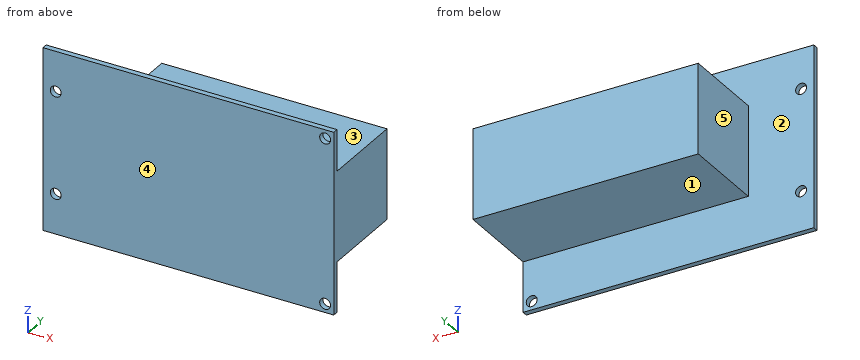
from build123d import *

# Parameters (mm, degrees)
SKETCH2_R           = 1.5
BOSS_EXTRUDE1_DEPTH = 1.5
SKETCH2_3_W         = 61.970625282
SKETCH2_3_H         = 24.8
BOSS_EXTRUDE2_DEPTH = 25


with BuildPart() as part:
    # Sketch2 → Boss-Extrude1 (new body)
    with BuildSketch(Plane(origin=(0, 0, 0), x_dir=(1, 0, 0), z_dir=(0, 1, 0))):
        Polygon((80, 0), (0, 0), (0, -50), (80, -50), (80, -38.6), (18.029374718, -38.6), (18.029374718, -13.8), (80, -13.8), align=None)
        with Locations((3.5, -39)):
            Circle(SKETCH2_R, mode=Mode.SUBTRACT)
        with Locations((77.62, -47.62)):
            Circle(SKETCH2_R, mode=Mode.SUBTRACT)
        with Locations((3.5, -11)):
            Circle(SKETCH2_R, mode=Mode.SUBTRACT)
        with Locations((77.62, -2.38)):
            Circle(SKETCH2_R, mode=Mode.SUBTRACT)
    extrude(amount=BOSS_EXTRUDE1_DEPTH)

    # Sketch2<3> → Boss-Extrude2 (add)
    with BuildSketch(Plane(origin=(0, 0, 0), x_dir=(1, 0, 0), z_dir=(0, 1, 0))):
        with Locations((49.014687359, -26.2)):
            Rectangle(SKETCH2_3_W, SKETCH2_3_H)
    extrude(amount=BOSS_EXTRUDE2_DEPTH)


solid = part.part
The listing builds one solid part. Answer for the finished solid, in the listing's coordinates (mm). Face numbers are marked on the shaded views. A direction names the side the tool comes from. Round coordinates to 2 decimals unless told otherwise and drop trailing zeros. Order: outer loops, then holes, each group sorted by start corner. A loop starts at its lowest first (then second) coordinate and runs counter-clockwise, first axis right, second up. Notation, with made-up numbers: M -10,36.5 L 11,36.5 A12 ccw 11,58.5 Z; hole C 66,83 d9. An arc over 180 degrees is marked long. Answer in a Markdown table with one row per item. Add a question column.
1) The part is cut by section C-C on z = 34. Determine the outline of the cut face in (x, y), plus the area to 3 significant figures.
2) The part is cut by section D-D on x = 51. Determine the outline of the cut face in (y, z), plus the area to 3 significant figures.
3) Determine the mould class of the marked faces 1, 2 and 3 for opening direction Z: pulls with the +Z half, pulls with the -Z half, needs draft (parallel to the pull), parting line crosses it, or undercut.
4) The part is cut by section A-A on x = 77.62. Determine the outline of the cut face in (y, z), plus the area to 3 significant figures.
5) The part is cut by section B-B on z = 47.62. Determine the outline of the cut face in (x, y), plus the area to 4 significant figures.
6) Consider line 1 along Z through (x, y) = (77.62, 0.9); line 2 along Z through (x, y) = (3.5, 1); line 3 along X through (y, z) = (0.6, 11). Determine where each line is inside the solid, lowest interval first. Write a range as from..to.
7) Flat-ended cylindrical pins translate along their axes: pin 1 Ø3.5 at (x, z) = (3.5, 39) entering from +Y; pin 2 Ø12 at (x, y) = (45, 11) entering from -Z; pin 3 Ø12 at (y, z) = (15.5, 21) entering from -X. Find the tip coordinate at first contact, or state that the pin passes through.
8) Which of the six approach directions +Z, -Z, +X, -X, +Y, -Y give full straight-line access (tool end or side, diameter ignored) to the marked faces 4 and 5?
Findings below:
| question | item | result |
|---|---|---|
| 1 | outline | M 0,0 L 80,0 L 80,25 L 18.03,25 L 18.03,1.5 L 0,1.5 Z |
| 1 | area | 1,580 mm² |
| 2 | outline | M 0,0 L 1.5,0 L 1.5,13.8 L 25,13.8 L 25,38.6 L 1.5,38.6 L 1.5,50 L 0,50 Z |
| 2 | area | 658 mm² |
| 3 | face 1 | pulls with the -Z half |
| 3 | face 2 | needs draft |
| 3 | face 3 | pulls with the +Z half |
| 4 | outline | M 0,0 L 1.5,0 L 1.5,0.88 L 0,0.88 Z; M 0,3.88 L 1.5,3.88 L 1.5,13.8 L 25,13.8 L 25,38.6 L 1.5,38.6 L 1.5,46.12 L 0,46.12 Z; M 0,49.12 L 1.5,49.12 L 1.5,50 L 0,50 Z |
| 4 | area | 649 mm² |
| 5 | outline | M 0,0 L 76.12,0 L 76.12,1.5 L 0,1.5 Z; M 79.12,0 L 80,0 L 80,1.5 L 79.12,1.5 Z |
| 5 | area | 115.5 mm² |
| 6 | line 1 | z = 0..0.88, 3.88..46.12, 49.12..50 |
| 6 | line 2 | z = 0..9.5, 12.5..37.5, 40.5..50 |
| 6 | line 3 | x = 0..2, 5..80 |
| 7 | pin 1 | stops at y = 1.5 |
| 7 | pin 2 | stops at z = 13.8 |
| 7 | pin 3 | stops at x = 18.03 |
| 8 | face 4 | +Z, -Z, +X, -X, -Y |
| 8 | face 5 | +Z, -Z, -X, +Y |
